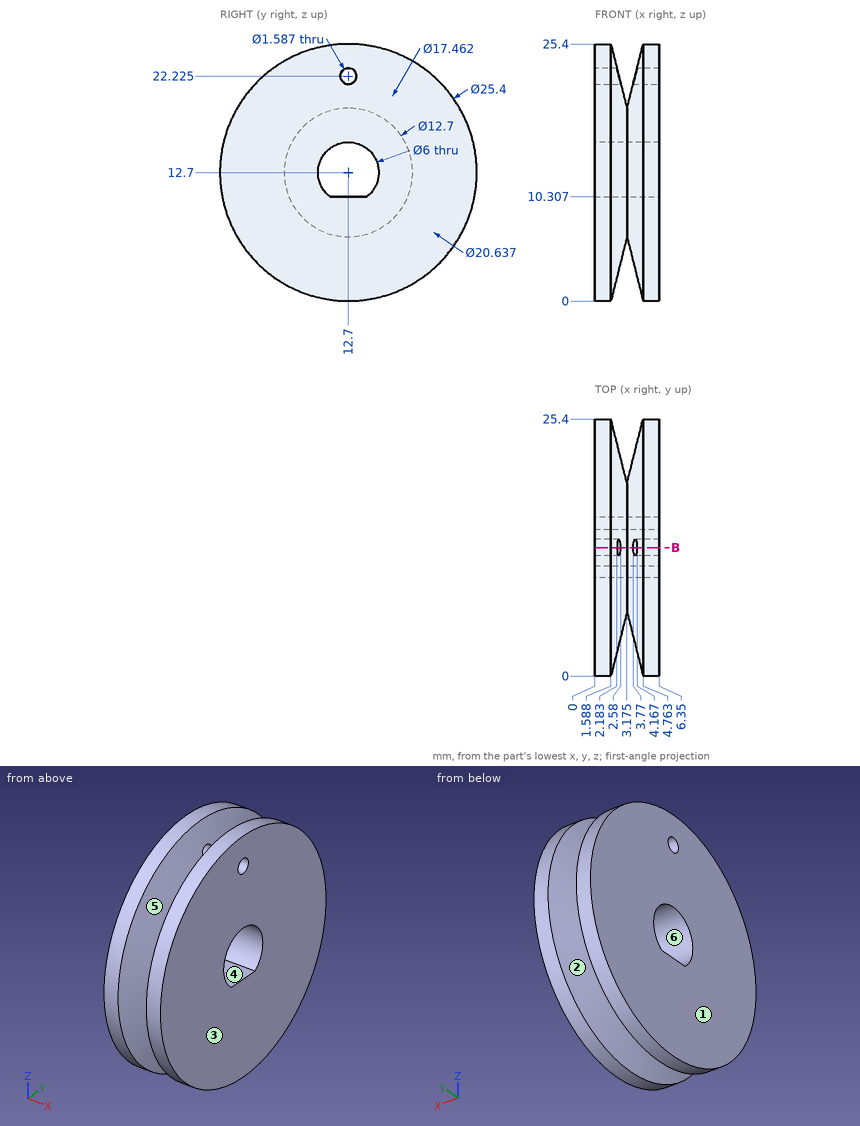
Could you check a few things on this drawing? It's one solid part, dimensions in mm from its lowest x, y, z. A direction names the side the tool comes from. Coordinates: 2 decimals unless noted, no trailing zeros. Put each result on its own line as item: value. Start each with the question number.
Q1. Which directions (+Z, -Z, +X, -X, +Y, -Y) give clear straight access to the entire face, cutting with the end or side of a thin tool? Please do the marked faces 5 and 6.
Q2. Thinking about a two-plate mould opening in X: for the marked faces 1, 2, 3 and 4, which applies, pulls with the +X half, pulls with the -X half, needs draft (parallel to the pull), parting line crosses it, or undercut?
Q3. I want a section at B-B on y = 12.7. Count the separate pieces of the cut face and the enclosed holes in it.
Q4. I'm going to push flat-ended pins straight in: P1, Ø2, axis at x = 4, y = 6, coming from the -Z side (1 decimal); P2, Ø3, axis at x = 4, z = 14, coming from the -Y side; P3, Ø1, axis at x = 2, z = 6.5, coming from the +Y side; P4, Ø1, axis at x = 1.5, y = 15.5, coming from the +Z side. Where does each tip first touch, or does it pass through?
Q5. Please list where these lines run through material, in increasing order: L1, parallel to Z at x = 5.75, y = 15.25 (1 decimal); L2, parallel to X at y = 18, z = 2; L3, parallel to Z at x = 1, y = 10 (1 decimal).
Checks:
1. face 5: none
1. face 6: +X, -X
2. face 1: pulls with the -X half
2. face 2: undercut
2. face 3: pulls with the +X half
2. face 4: needs draft
3. separate pieces: 4
3. enclosed holes: 0
4. P1: z = 1.5
4. P2: y = 0
4. P3: y = 23.94
4. P4: z = 25.19
5. L1: 0.3 to 11.1, 14.3 to 25.1
5. L2: 0 to 1.78, 4.57 to 6.35
5. L3: 0.3 to 11.4, 14 to 25.1
